from build123d import *

# Parameters (mm, degrees)
BOSS_EXTRUDE1_DEPTH              = 13
CUT_EXTRUDE1_DEPTH               = 201.804739102
CUT_EXTRUDE2_DEPTH               = 201.804739102
CUT_EXTRUDE3_DEPTH               = 201.804739102
CUT_EXTRUDE4_DEPTH               = 201.804739102
CUT_EXTRUDE5_DEPTH               = 7.8
SKETCH9_W                        = 4.064
SKETCH9_H                        = 5.2
F_1_4_CLEARANCE_HOLE1_AT_2_COUNT = 2
F_1_4_CLEARANCE_HOLE1_AT_2_PITCH = 107.95
F_1_4_CLEARANCE_HOLE1_AT_3_COUNT = 2
F_1_4_CLEARANCE_HOLE1_AT_3_PITCH = 186.974884677
F_1_4_CLEARANCE_HOLE1_AT_4_COUNT = 2
F_1_4_CLEARANCE_HOLE1_AT_4_PITCH = 215.9
F_1_4_CLEARANCE_HOLE1_AT_5_COUNT = 2
F_1_4_CLEARANCE_HOLE1_AT_5_PITCH = 107.95
HOLE1_D                          = 6.3
HOLE2_D                          = 101.44
F_8_CLEARANCE_HOLE1_D            = 4.88
CIRPATTERN2_COUNT                = 6


with BuildPart() as part:
    # Sketch1 → Boss-Extrude1 (new body)
    with BuildSketch(Plane(origin=(0, 0, 0), x_dir=(1, 0, 0), z_dir=(0, 1, 0))):
        with BuildLine():
            Line((164.38099488, 61.17), (96.905432604, 61.17))
            ThreePointArc((96.905432604, 61.17), (-114.596822679, 0), (96.905432604, -61.17))
            Line((96.905432604, -61.17), (164.38099488, -61.17))
            Line((164.38099488, -61.17), (164.38099488, 61.17))
        make_face()
    extrude(amount=-BOSS_EXTRUDE1_DEPTH)

    # Sketch2 → Cut-Extrude1 (cut, through all)
    with BuildSketch(Plane.XZ.offset(13)):
        with BuildLine():
            ThreePointArc((36.664399822, -63.490820086), (33.280235587, -76.125443336), (45.914858837, -79.509607572))
            ThreePointArc((45.914858837, -79.509607572), (65.250493783, -64.593536978), (79.970145175, -45.107957601))
            ThreePointArc((79.970145175, -45.107957601), (76.458305593, -32.508225263), (63.858573255, -36.020064845))
            ThreePointArc((63.858573255, -36.020064845), (52.104487594, -51.579887768), (36.664399822, -63.490820086))
        make_face()
    extrude(amount=-CUT_EXTRUDE1_DEPTH, mode=Mode.SUBTRACT)

    # Sketch3 → Cut-Extrude2 (cut, through all)
    with BuildSketch(Plane.XZ.offset(13)):
        with BuildLine():
            ThreePointArc((45.914858837, 79.509607572), (33.280235587, 76.125443336), (36.664399822, 63.490820086))
            ThreePointArc((36.664399822, 63.490820086), (52.104487594, 51.579887768), (63.858573255, 36.020064845))
            ThreePointArc((63.858573255, 36.020064845), (76.458305593, 32.508225263), (79.970145175, 45.107957601))
            ThreePointArc((79.970145175, 45.107957601), (65.250493783, 64.593536978), (45.914858837, 79.509607572))
        make_face()
    extrude(amount=-CUT_EXTRUDE2_DEPTH, mode=Mode.SUBTRACT)

    # Sketch4 → Cut-Extrude3 (cut, through all)
    with BuildSketch(Plane.XZ.offset(13)):
        with BuildLine():
            ThreePointArc((-12.00973997, -91.025919957), (-4.095291585, -82.854974293), (-9.276109056, -72.727685583))
            ThreePointArc((-9.276109056, -72.727685583), (-48.237079471, -55.213645176), (-70.823685709, -18.957003774))
            ThreePointArc((-70.823685709, -18.957003774), (-82.149557569, -12.413999964), (-88.692561379, -23.739871823))
            ThreePointArc((-88.692561379, -23.739871823), (-60.556514452, -69.01348068), (-12.00973997, -91.025919957))
        make_face()
    extrude(amount=-CUT_EXTRUDE3_DEPTH, mode=Mode.SUBTRACT)

    # Sketch5 → Cut-Extrude4 (cut, through all)
    with BuildSketch(Plane.XZ.offset(13)):
        with BuildLine():
            ThreePointArc((-88.692561379, 23.739871823), (-82.149557569, 12.413999964), (-70.823685709, 18.957003774))
            ThreePointArc((-70.823685709, 18.957003774), (-48.237079471, 55.213645176), (-9.276109056, 72.727685583))
            ThreePointArc((-9.276109056, 72.727685583), (-4.095291585, 82.854974293), (-12.00973997, 91.025919957))
            ThreePointArc((-12.00973997, 91.025919957), (-60.556514452, 69.01348068), (-88.692561379, 23.739871823))
        make_face()
    extrude(amount=-CUT_EXTRUDE4_DEPTH, mode=Mode.SUBTRACT)

    # Sketch6 → Cut-Extrude5 (cut)
    with BuildSketch(Plane(origin=(0, 0, 0), x_dir=(-1, 0, 0), z_dir=(0, 1, 0))):
        with BuildLine():
            Line((114.362561544, 7.323679763), (106.996209034, 7.342768071))
            ThreePointArc((106.996209034, 7.342768071), (99.356489103, -0.257460832), (106.956718006, -7.897180763))
            Line((106.956718006, -7.897180763), (114.323070516, -7.91626907))
            ThreePointArc((114.323070516, -7.91626907), (114.596437937, -0.29695186), (114.362561544, 7.323679763))
        make_face()
    cut_extrude5 = extrude(amount=-CUT_EXTRUDE5_DEPTH, mode=Mode.SUBTRACT)

    # Sketch9 → 1/4 Clearance Hole1 (revolve, cut)
    with BuildSketch(Plane(origin=(-53.975, -7.8, 93.487442339), x_dir=(0, 0, 1), z_dir=(1, 0, 0))):
        with Locations((2.032, 2.6)):
            Rectangle(SKETCH9_W, SKETCH9_H)
    f_1_4_clearance_hole1 = revolve(axis=Axis((-53.975, -1.45, 93.487442339), (0, -1, 0)), mode=Mode.SUBTRACT)

    # 1/4 Clearance Hole1 at 2: 1/4 Clearance Hole1 ×2
    with Locations(*[Vector(-0.499999999999995, 0, -0.8660254037844416) * (i * F_1_4_CLEARANCE_HOLE1_AT_2_PITCH) for i in range(1, F_1_4_CLEARANCE_HOLE1_AT_2_COUNT)]):
        add(f_1_4_clearance_hole1, mode=Mode.SUBTRACT)

    # 1/4 Clearance Hole1 at 3: 1/4 Clearance Hole1 ×2
    with Locations(*[(0, 0, -i * F_1_4_CLEARANCE_HOLE1_AT_3_PITCH) for i in range(1, F_1_4_CLEARANCE_HOLE1_AT_3_COUNT)]):
        add(f_1_4_clearance_hole1, mode=Mode.SUBTRACT)

    # 1/4 Clearance Hole1 at 4: 1/4 Clearance Hole1 ×2
    with Locations(*[Vector(0.5000000000000071, 0, -0.8660254037844346) * (i * F_1_4_CLEARANCE_HOLE1_AT_4_PITCH) for i in range(1, F_1_4_CLEARANCE_HOLE1_AT_4_COUNT)]):
        add(f_1_4_clearance_hole1, mode=Mode.SUBTRACT)

    # 1/4 Clearance Hole1 at 5: 1/4 Clearance Hole1 ×2
    with Locations(*[(i * F_1_4_CLEARANCE_HOLE1_AT_5_PITCH, 0, 0) for i in range(1, F_1_4_CLEARANCE_HOLE1_AT_5_COUNT)]):
        add(f_1_4_clearance_hole1, mode=Mode.SUBTRACT)

    # Hole1 (through all)
    with Locations(Plane(origin=(0, 0, 0), x_dir=(1, 0, 0), z_dir=(0, 1, 0))):
        with Locations((63.27, 0), (0, -63.27), (-63.27, 0), (0, 63.27)):
            Hole(HOLE1_D / 2)

    # Hole2 (through all)
    with Locations(Plane(origin=(0, 0, 0), x_dir=(1, 0, 0), z_dir=(0, 1, 0))):
        with Locations((0, 0)):
            Hole(HOLE2_D / 2)

    # #8 Clearance Hole1 (through all)
    with Locations(Plane(origin=(0, -13, 0), x_dir=(-1, 0, 0), z_dir=(0, -1, 0))):
        with Locations((-159.64099488, -40.668301559), (-159.64099488, 17.964494153), (-126.578871671, 57.63), (-126.578871671, -57.63), (-159.64099488, 43.162614752), (-159.64099488, -15.500531602), (-100.720889468, 57.63), (-100.720889468, -57.63)):
            Hole(F_8_CLEARANCE_HOLE1_D / 2)

    # CirPattern2: Cut-Extrude5 ×6 about axis, 1 skipped
    cirpattern2_axis = Axis((0, 0, 0), (0, 1, 0))
    add([cut_extrude5.rotate(cirpattern2_axis, i * 360 / CIRPATTERN2_COUNT) for i in range(1, CIRPATTERN2_COUNT) if i not in (3,)], mode=Mode.SUBTRACT)


solid = part.part
Geometry: final body of the model. Coordinates: model frame, mm. A direction names the side the tool comes from. Coordinates: 2 decimals unless noted, no trailing zeros. Order: outer loops, then holes, each group sorted by start corner. A loop starts at its lowest first (then second) coordinate and runs counter-clockwise, first axis right, second up.
1) Set-up query: faces 1 (the flat face through (-105, -7.8, -4)), 2 (the flat face through (48.45, -3.85, 99.73)), 3 (the flat face through (62.14, -3.85, -91.82)), 4 (the cylindrical face through (-4.072, -6.591, 82.687)). Return all of +Z, -Z, +X, -X, +Y, -Y with unobstructed straight access to the full face (end or side cutting, diameter ignored); none if empty.
Result sheet:
face 1: -X, +Y
face 2: +X, +Y
face 3: -Z, +Y
face 4: +Y, -Y
2) Section D-D (x = -32). Return loops of the section in (y, z).
Result sheet:
outline: (-13, -110.04) - (0, -110.04) - (0, -86.06) - (-13, -86.06) - close; (-13, -65.96) - (0, -65.96) - (0, -39.35) - (-13, -39.35) - close; (-13, 39.35) - (0, 39.35) - (0, 65.96) - (-13, 65.96) - close; (-13, 86.06) - (0, 86.06) - (0, 110.04) - (-13, 110.04) - close
3) Section A-A (x = 0). Return loops of the section in (y, z).
Result sheet:
outline: (-13, -114.6) - (0, -114.6) - (0, -66.42) - (-13, -66.42) - close; (-13, -60.12) - (0, -60.12) - (0, -50.72) - (-13, -50.72) - close; (-13, 50.72) - (0, 50.72) - (0, 60.12) - (-13, 60.12) - close; (-13, 66.42) - (0, 66.42) - (0, 114.6) - (-13, 114.6) - close
4) First-contact query: P1, Ø4, axis at x = -76.5, y = -3, coming from the +Z side; P2, Ø1, axis at x = 56, y = -2.5, coming from the -Z side; P3, Ø5, axis at y = -11.5, z = 79, coming from the -X side. Flat tips, straight axial feed; report the tip coordinate or a pass-through.
Result sheet:
P1: stops at z = 87.08
P2: stops at z = -85.41
P3: stops at x = -85.32
5) Draft query along Z for faces 5 (the cylindrical face through (40.25, -6.59, 30.86)), 6 (the flat face through (54, 0, -2)), 7 (the flat face through (131, -6, -61.17)). Return one class per face: released by +Z, released by -Z, zero draft, split by the parting line, or undercut.
Result sheet:
face 5: undercut
face 6: zero draft
face 7: released by -Z
6) Section B-B (z = 0). Return loops of the section in (x, y).
Result sheet:
outline: (-114.6, -13) - (-112.01, -13) - (-112.01, -7.8) - (-114.6, -7.8) - close; (-103.89, -13) - (-66.42, -13) - (-66.42, 0) - (-99.36, 0) - (-99.36, -7.8) - (-103.89, -7.8) - close; (-60.12, -13) - (-50.72, -13) - (-50.72, 0) - (-60.12, 0) - close; (50.72, -13) - (60.12, -13) - (60.12, 0) - (50.72, 0) - close; (66.42, -13) - (164.38, -13) - (164.38, 0) - (66.42, 0) - close
7) Section C-C (x = -81). Return loops of the section in (y, z).
Result sheet:
outline: (-13, -81.06) - (0, -81.06) - (0, -43.23) - (-13, -43.23) - close; (-13, -12.18) - (0, -12.18) - (0, 12.18) - (-13, 12.18) - close; (-13, 43.23) - (0, 43.23) - (0, 81.06) - (-13, 81.06) - close
8) Ray query, probe 1 along Z at (x, y) = (-1, -8.25); probe 2 along X at (y, z) = (-11, -62.5); probe 3 along X at (y, z) = (-6.5, -20.5). Return the intervals inside material, ascending.
Result sheet:
probe 1: z = -114.59 to -66.26, -60.28 to -50.71, 50.71 to 60.28, 66.26 to 114.59
probe 2: x = -96.05 to -67.26, -38.33 to -3.05, 3.05 to 38.33, 67.26 to 96.05
probe 3: x = -112.75 to -88.97, -70.39 to -46.39, 46.39 to 164.38
